Geometry check sheet. Reference: the model listing, model coordinates, mm. A direction names the side the tool comes from. Coordinates: 2 decimals unless noted, no trailing zeros. Write each loop counter-clockwise with the first axis right and the second up, starting at its lowest first coordinate (ties: lowest second). Pieces come first, ordered by that corner, then holes. Notation, with made-up numbers: (50.25, 38.25) -> (107.25, 38.25) arc R15 ccw to (107.25, 43.25) -> close; hole circle Ø4 at (-12, -13). An arc over 180 degrees is marked (long way). One line per question, with ' | ' between items.
```python
from build123d import *

# Parameters (mm, degrees)
SKETCH_1_R                = 1.7
EXTRUDE_6_DEPTH           = 4
EXTRUDE_7_DEPTH           = 100
SKETCH_10_W               = 140
SKETCH_10_H               = 96
CUT_EXTRUDE_20_DEPTH      = 115
CUT_EXTRUDE_22_DEPTH      = 220.402235989
CUT_EXTRUDE_22_DEPTH_BACK = 220.402235989
SKETCH_16_R               = 1.5
SKETCH_16_R_2             = 4
SKETCH_21_W               = 110
SKETCH_21_H               = 80
CUT_EXTRUDE_28_DEPTH      = 50
SKETCH_23_R               = 5
CUT_EXTRUDE_29_DEPTH      = 220.402235989
SKETCH_22_W               = 148
SKETCH_22_H               = 104
SKETCH_22_W_2             = 144
SKETCH_22_H_2             = 100
EXTRUDE_8_DEPTH           = 10
CUT_EXTRUDE_30_DEPTH      = 177.910545635
CUT_EXTRUDE_30_DEPTH_BACK = 177.910545635
SKETCH_27_R               = 2
CUT_EXTRUDE_31_DEPTH      = 219.058114174
CUT_EXTRUDE_31_DEPTH_BACK = 219.058114174
SKETCH_30_R               = 2


with BuildPart() as part:
    # 草图1 → 凸台-拉伸6 (new body)
    with BuildSketch(Plane(origin=(0, 0, 0), x_dir=(1, 0, 0), z_dir=(0, 1, 0))):
        with BuildLine():
            Line((-74, 0), (-74, -115))
            ThreePointArc((-74, -115), (-71.363961031, -121.363961031), (-65, -124))
            Line((-65, -124), (65, -124))
            ThreePointArc((65, -124), (71.363961031, -121.363961031), (74, -115))
            Line((74, -115), (74, 0))
            Line((74, 0), (-74, 0))
        make_face()
        with Locations(Location((-62, -108, 0), (0, 0, 270))):
            Circle(SKETCH_1_R, mode=Mode.SUBTRACT)
        with Locations(Location((-48, -108, 0), (0, 0, 270))):
            Circle(SKETCH_1_R, mode=Mode.SUBTRACT)
        with Locations(Location((48, -108, 0), (0, 0, 270))):
            Circle(SKETCH_1_R, mode=Mode.SUBTRACT)
        with Locations(Location((62, -108, 0), (0, 0, 270))):
            Circle(SKETCH_1_R, mode=Mode.SUBTRACT)
        with Locations(Location((-62, -92, 0), (0, 0, 270))):
            Circle(SKETCH_1_R, mode=Mode.SUBTRACT)
        with Locations(Location((-48, -92, 0), (0, 0, 270))):
            Circle(SKETCH_1_R, mode=Mode.SUBTRACT)
        with BuildLine():
            ThreePointArc((-25, -90), (-23.535533906, -86.464466094), (-20, -85))
            Line((-20, -85), (20, -85))
            ThreePointArc((20, -85), (23.535533906, -86.464466094), (25, -90))
            Line((25, -90), (25, -107.989151936))
            ThreePointArc((25, -107.989151936), (23.535533906, -111.524685842), (20, -112.989151936))
            Line((20, -112.989151936), (-20, -112.989151936))
            ThreePointArc((-20, -112.989151936), (-23.535533906, -111.524685842), (-25, -107.989151936))
            Line((-25, -107.989151936), (-25, -90))
        make_face(mode=Mode.SUBTRACT)
        with Locations(Location((48, -92, 0), (0, 0, 270))):
            Circle(SKETCH_1_R, mode=Mode.SUBTRACT)
        with Locations(Location((62, -92, 0), (0, 0, 270))):
            Circle(SKETCH_1_R, mode=Mode.SUBTRACT)
    extrude(amount=EXTRUDE_6_DEPTH)

    # 草图9 → 凸台-拉伸7 (add)
    with BuildSketch(Plane(origin=(0, 4, 0), x_dir=(1, 0, 0), z_dir=(0, 1, 0))):
        with BuildLine():
            Line((-74, 0), (74, 0))
            Line((74, 0), (74, -115.166586314))
            ThreePointArc((74, -115.166586314), (71.363961031, -121.530547345), (65, -124.166586314))
            Line((65, -124.166586314), (-65, -124.166586314))
            ThreePointArc((-65, -124.166586314), (-71.363961031, -121.530547345), (-74, -115.166586314))
            Line((-74, -115.166586314), (-74, 0))
        make_face()
    extrude(amount=EXTRUDE_7_DEPTH)

    # 草图10 → 切除-拉伸20 (cut)
    with BuildSketch(Plane(origin=(0, 0, 0), x_dir=(-1, 0, 0), z_dir=(0, 0, -1))):
        with Locations((0, 52)):
            Rectangle(SKETCH_10_W, SKETCH_10_H)
    extrude(amount=-CUT_EXTRUDE_20_DEPTH, mode=Mode.SUBTRACT)

    # 草图16 → 切除-拉伸22 (cut, two sides: drawn at the far end of the back side and taken through both)
    with BuildSketch(Plane.ZY.offset(74).offset(-CUT_EXTRUDE_22_DEPTH_BACK)):
        with Locations(Location((100, 16.25, 0), (0, 0, 180))):
            Circle(SKETCH_16_R)
        with Locations(Location((108.5, 24.75, 0), (0, 0, 180))):
            Circle(SKETCH_16_R)
        with Locations(Location((100, 24.75, 0), (0, 0, 180))):
            Circle(SKETCH_16_R_2)
        with Locations(Location((91.5, 24.75, 0), (0, 0, 180))):
            Circle(SKETCH_16_R)
        with Locations(Location((100, 33.25, 0), (0, 0, 180))):
            Circle(SKETCH_16_R)
    extrude(amount=CUT_EXTRUDE_22_DEPTH + CUT_EXTRUDE_22_DEPTH_BACK, mode=Mode.SUBTRACT)

    # 草图21 → 切除-拉伸28 (cut)
    with BuildSketch(Plane.XY.offset(124.166586314)):
        with Locations((0, 54)):
            Rectangle(SKETCH_21_W, SKETCH_21_H)
    extrude(amount=-CUT_EXTRUDE_28_DEPTH, mode=Mode.SUBTRACT)

    # 草图23 → 切除-拉伸29 (cut, through all)
    with BuildSketch(Plane.ZY.offset(74)):
        with Locations((100, 24.75)):
            Circle(SKETCH_23_R)
    extrude(amount=-CUT_EXTRUDE_29_DEPTH, mode=Mode.SUBTRACT)

    # 草图22 → 凸台-拉伸8 (add)
    with BuildSketch(Plane(origin=(0, 0, 0), x_dir=(-1, 0, 0), z_dir=(0, 0, -1))):
        with Locations((0, 52)):
            Rectangle(SKETCH_22_W, SKETCH_22_H)
        with Locations((0, 52)):
            Rectangle(SKETCH_22_W_2, SKETCH_22_H_2, mode=Mode.SUBTRACT)
    extrude(amount=EXTRUDE_8_DEPTH)

    # 草图27 → 切除-拉伸30 (cut, two sides: drawn at the far end of the back side and taken through both)
    with BuildSketch(Plane.XZ.offset(-102).offset(-CUT_EXTRUDE_30_DEPTH_BACK)):
        with Locations(Location((-60, -5, 0), (0, 0, 180))):
            Circle(SKETCH_27_R)
        with Locations(Location((-40, -5, 0), (0, 0, 180))):
            Circle(SKETCH_27_R)
        with Locations(Location((-20, -5, 0), (0, 0, 180))):
            Circle(SKETCH_27_R)
        with Locations(Location((40, -5, 0), (0, 0, 180))):
            Circle(SKETCH_27_R)
        with Locations(Location((0, -5, 0), (0, 0, 180))):
            Circle(SKETCH_27_R)
        with Locations(Location((20, -5, 0), (0, 0, 180))):
            Circle(SKETCH_27_R)
        with Locations(Location((60, -5, 0), (0, 0, 180))):
            Circle(SKETCH_27_R)
    extrude(amount=CUT_EXTRUDE_30_DEPTH + CUT_EXTRUDE_30_DEPTH_BACK, mode=Mode.SUBTRACT)

    # 草图30 → 切除-拉伸31 (cut, two sides: drawn at the far end of the back side and taken through both)
    with BuildSketch(Plane(origin=(-72, 0, 0), x_dir=(0, 0, -1), z_dir=(1, 0, 0)).offset(-CUT_EXTRUDE_31_DEPTH_BACK)):
        with Locations(Location((5, 52, 0), (0, 0, 90))):
            Circle(SKETCH_30_R)
        with Locations(Location((5, 72, 0), (0, 0, 90))):
            Circle(SKETCH_30_R)
        with Locations(Location((5, 92, 0), (0, 0, 90))):
            Circle(SKETCH_30_R)
        with Locations(Location((5, 12, 0), (0, 0, 90))):
            Circle(SKETCH_30_R)
        with Locations(Location((5, 32, 0), (0, 0, 90))):
            Circle(SKETCH_30_R)
    extrude(amount=CUT_EXTRUDE_31_DEPTH + CUT_EXTRUDE_31_DEPTH_BACK, mode=Mode.SUBTRACT)


solid = part.part
```
(1) Cross-section at A-A (y = 60). Record the cut outline in (x, z).
Answers below:
outline: (-74, -10) -> (-72, -10) -> (-72, 0) -> (-70, 0) -> (-70, 115) -> (-55, 115) -> (-55, 124.17) -> (-65, 124.17) arc R9 ccw to (-74, 115.17) -> close; (55, 115) -> (70, 115) -> (70, 0) -> (72, 0) -> (72, -10) -> (74, -10) -> (74, 115.17) arc R9 ccw to (65, 124.17) -> (55, 124.17) -> close
(2) Material ranges on line 1 (Y direction, x = -73.2, z = -5); line 2 (Y direction, x = 36.5, z = 14); line 3 (X direction, y = 2.05, z = 92), recorded low to high.
Answers below:
line 1: y = 0 to 10, 14 to 30, 34 to 50, 54 to 70, 74 to 90, 94 to 104 | line 2: y = 0 to 4, 100 to 104 | line 3: x = -74 to -63.7, -60.3 to -49.7, -46.3 to -25, 25 to 46.3, 49.7 to 60.3, 63.7 to 74
(3) Draft check along X on faces 1 (the face through (-71.294, 53.3, 121.6)), 2 (the face through (73, 10.4, -6.2)), 3 (the face through (1, 4, 57)). Enter one of: pulls with the +X half, pulls with the -X half, needs draft (parallel to the pull), parting line crosses it, or undercut.
Answers below:
face 1: pulls with the -X half | face 2: needs draft | face 3: undercut
(4) Tool access check on faces 4 (the face through (-1, 14, 120)), 5 (the face through (-47.93, 1.97, 106.3)), 6 (the face through (-1, 2, 124)), 7 (the face through (1, 100, 57)), 8 (the face through (-58, 1, -5)). Record the directions out of +Z, -Z, +X, -X, +Y, -Y that give a thin tool (end or side, any length) a straight path to the whole face; none if there is none.
Answers below:
face 4: +Z, -Z | face 5: -Y | face 6: +Z, +X, -X, -Y | face 7: -Z | face 8: +Y, -Y
(5) Depth check by flat-ended pin: P1, Ø2.5, axis at y = 33.25, z = 100, coming from the -X side; P2, Ø3, axis at x = -48, z = 108, coming from the -Y side; P3, Ø4.5, axis at y = 74, z = 118, coming from the -X side. Enter the tip coordinate at first touch or a pass-through.
Answers below:
P1: passes through | P2: stops at y = 100 | P3: stops at x = -73.98
(6) Cross-section at B-B (z = 74). Record the cut outline in (x, y).
Answers below:
outline: (-74, 0) -> (74, 0) -> (74, 104) -> (-74, 104) -> close; hole (-70, 4) -> (70, 4) -> (70, 100) -> (-70, 100) -> close
(7) Cross-section at C-C (x = -40). Record the cut outline in (y, z), plus the area to 3 significant figures.
Answers below:
outline: (0, -10) -> (2, -10) -> (2, -7) -> (0, -7) -> close; (0, -3) -> (2, -3) -> (2, 0) -> (4, 0) -> (4, 115) -> (14, 115) -> (14, 124.17) -> (4, 124.17) -> (4, 124) -> (0, 124) -> close; (94, 115) -> (100, 115) -> (100, 0) -> (102, 0) -> (102, -3) -> (104, -3) -> (104, 124.17) -> (94, 124.17) -> close; (102, -10) -> (104, -10) -> (104, -7) -> (102, -7) -> close | area: 1,160 mm²
